```python
from build123d import *

# Parameters (mm, degrees)
F0_R     = 5
F1_DEPTH = 5
F2_R     = 2.25
F3_DEPTH = 10
F5_DEPTH = 2


with BuildPart() as f1:
    # F0 (on Right) → F1 (new body)
    with BuildSketch(Plane.YZ):
        Circle(F0_R)
    extrude(amount=F1_DEPTH)

    # F2 (on face) → F3 (join)
    with BuildSketch(Plane(origin=(0, 0, 0), x_dir=(0, -1, 0), z_dir=(-1, 0, 0))):
        Circle(F2_R)
    extrude(amount=F3_DEPTH)

    # F4 (on face) → F5 (cut)
    with BuildSketch(Plane.YZ.offset(5)):
        with BuildLine():
            Line((0.4713461094, 4.9777337057), (0.4713461094, 6.4907008782))
            Line((0.4713461094, 6.4907008782), (-0.4713461094, 6.4907008782))
            Line((-0.4713461094, 6.4907008782), (-0.4713461094, 4.9777337057))
            ThreePointArc((-0.4713461094, 4.9777337057), (0, 5), (0.4713461094, 4.9777337057))
        make_face()
        with BuildLine():
            Line((0.4713461094, -4.9777337057), (0.4713461094, 4.9777337057))
            ThreePointArc((0.4713461094, 4.9777337057), (0, 5), (-0.4713461094, 4.9777337057))
            Line((-0.4713461094, 4.9777337057), (-0.4713461094, -4.9777337057))
            ThreePointArc((-0.4713461094, -4.9777337057), (0, -5), (0.4713461094, -4.9777337057))
        make_face()
        with BuildLine():
            Line((0.4713461094, -6.4907008782), (0.4713461094, -4.9777337057))
            ThreePointArc((0.4713461094, -4.9777337057), (0, -5), (-0.4713461094, -4.9777337057))
            Line((-0.4713461094, -4.9777337057), (-0.4713461094, -6.4907008782))
            Line((-0.4713461094, -6.4907008782), (0.4713461094, -6.4907008782))
        make_face()
    extrude(amount=-F5_DEPTH, mode=Mode.SUBTRACT)


solid = f1.part
```
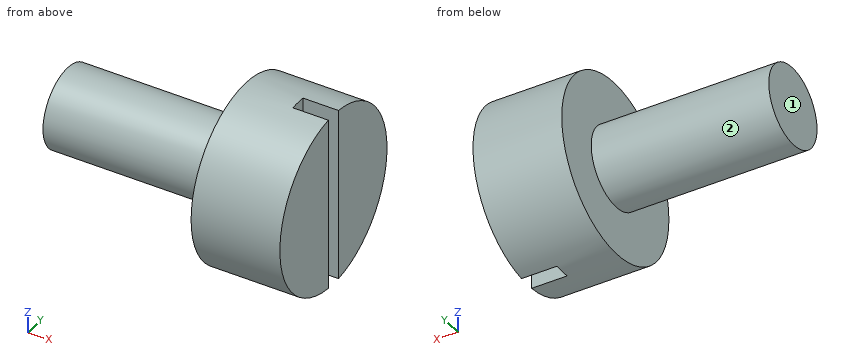
Can you work these out from the model? Positions are in its coordinate system, mm. Face numbers are marked on the shaded views. A direction names the side the tool comes from. Give positions to 0.01 mm unless a question says otherwise; leave off trailing zeros. Loops run counter-clockwise (first coordinate to the right, second up) from the corner with the lowest first, then second, coordinate; pieces in that order, holes last. Notation, with made-up numbers: M 52.25,53.5 L 83.25,53.5 A17 ccw 83.25,66.5 Z; hole C -5.5,34.25 d5. An arc over 180 degrees is marked long. Use one line per item in the form item = value. Start each with the question number.
(1) I want a section at D-D, the plane x = 1.5. Write out the boundary of the cut face in (y, z), and give its area (3 significant figures).
(2) I want a section at A-A, the plane y = 0. Write out the boundary of the cut face in (x, z).
(3) Please list where these lines run through material, in increasing order: line 1 (X direction, y = 0, z = 2); line 2 (X direction, y = -3, z = -3.25); line 3 (Y direction, x = 3.75, z = -2).
(4) I want a section at B-B, the plane z = -3. Write out the boundary of the cut face in (x, y).
(5) I'm going to push flat-ended pins straight in: P1, Ø0.8, axis at y = 0, z = 0, coming from the +X side; P2, Ø1.5, axis at x = -3.5, z = 1, coming from the -Y side; P3, Ø2, axis at x = 2, y = -0.5, coming from the -Z side; P4, Ø2, axis at x = 0.5, z = 3.5, coming from the +Y side. Where does each tip first touch, or does it pass through?
(6) I want a section at C-C, the plane x = 3.5. Write out the boundary of the cut face in (y, z).
(7) On a 3-axis mill with a long thin cutter (end or side, diameter ignored), from which of +Z, -Z, +X, -X, +Y, -Y can I reach the whole of each face in a straight line? I mean the marked faces 1 and 2. Say none if no direction works.
Worked out:
q1.outline = C 0,0 d10
q1.area = 78.5 mm²
q2.outline = M -10,-2.25 L 0,-2.25 L 0,-5 L 3,-5 L 3,5 L 0,5 L 0,2.25 L -10,2.25 Z
q3.line_1 = -10 to 3
q3.line_2 = 0 to 5
q3.line_3 = -4.58 to -0.47, 0.47 to 4.58
q4.outline = M 0,-4 L 5,-4 L 5,-0.47 L 3,-0.47 L 3,0.47 L 5,0.47 L 5,4 L 0,4 Z
q5.P1 = 3
q5.P2 = -2.24
q5.P3 = -5
q5.P4 = 4.33
q6.outline = M -0.47,-4.98 L -0.47,4.98 A5 ccw Z; M 0.47,-4.98 A5 ccw 0.47,4.98 Z
q7.face_1 = +Z, -Z, -X, +Y, -Y
q7.face_2 = -X
